Check sheet for the modelled part. Datum: model origin and axes. Units: mm. Round coordinates to 2 decimals unless told otherwise and drop trailing zeros. Order: outer loops, then holes, each group sorted by start corner. A loop starts at its lowest first (then second) coordinate and runs counter-clockwise, first axis right, second up. Notation, with made-up numbers: (64, 78) -> (82, 78) arc R23 cw to (82, 117) -> close; hole circle Ø1 at (-23, 22.25). An arc over 180 degrees is marked (long way). Answer in a Markdown table with one row per item.
```python
from build123d import *

# Parameters (mm, degrees)
FILLET1_R           = 2
FILLET2_R           = 10
SKETCH3_W           = 10
SKETCH3_H           = 20
BOSS_EXTRUDE1_DEPTH = 25
BOSS_EXTRUDE2_REACH = 322.147
SKETCH4_W           = 50
SKETCH4_H           = 20


with BuildPart() as part:
    # Sketch1 → Revolve1 (revolve)
    with BuildSketch(Plane.XY):
        Polygon((0, 0), (150, 0), (50, 100), (25, 100), (25, 50), (0, 50), align=None)
    revolve(axis=Axis((0, 50, 0), (0, -1, 0)))

    # Fillet1
    fillet1_edges = [part.edges().sort_by_distance(p)[0] for p in [
        (-25, 100, 0),
        (-50, 100, 0),
    ]]
    fillet(fillet1_edges, radius=FILLET1_R)

    # Fillet2
    fillet2_edges = [part.edges().sort_by_distance(p)[0] for p in [
        (-150, 0, 0),
    ]]
    fillet(fillet2_edges, radius=FILLET2_R)

    # Sketch4 → Boss-Extrude2 (add, up to next)
    with BuildSketch(Plane(origin=(-136.238585348, 0, 0), x_dir=(0, 0, -1), z_dir=(1, 0, 0)), mode=Mode.PRIVATE) as boss_extrude2_sk1:
        with Locations((0, 15)):
            Rectangle(SKETCH4_W, SKETCH4_H)
    boss_extrude2_tool1 = extrude(boss_extrude2_sk1.sketch, amount=BOSS_EXTRUDE2_REACH, mode=Mode.PRIVATE) - part.part


with BuildPart() as body_2:
    # Sketch3 → Boss-Extrude1 (new, symmetric)
    with BuildSketch(Plane.XY):
        with Locations((-141.238585348, 15)):
            Rectangle(SKETCH3_W, SKETCH3_H)
    extrude(amount=BOSS_EXTRUDE1_DEPTH, both=True)


with BuildPart() as part_1:
    add(part.part)

    add(body_2.part)  # Boss-Extrude2 merges body 2
    add(boss_extrude2_tool1.solids().sort_by_distance((-136.238585, 15, 0))[0])


solid = part_1.part
```
(1) Draft check along X on faces 1 (the flat face through (0, 50, 0)), 2 (the conical face through (52.06, 95.42, 16.4)), 3 (the cylindrical face through (23.846, 73.664, 7.509)), 4 (the flat face through (-139, 5, 0)). Enter one of: pulls with the +X half, pulls with the -X half, needs draft (parallel to the pull), parting line crosses it, or undercut.
Solutions:
| item | result |
|---|---|
| face 1 | undercut |
| face 2 | parting line crosses it |
| face 3 | undercut |
| face 4 | needs draft |
(2) Section check D-D on y = 83. Record the boundary of the cut face in (x, z).
Solutions:
| item | result |
|---|---|
| outline | circle Ø134 at (0, 0); hole circle Ø50 at (0, 0) |
(3) Section check B-B on z = 0. Record the boundary of the cut face in (x, y).
Solutions:
| item | result |
|---|---|
| outline | (-146.24, 5) -> (-134.52, 5) arc R10 ccw to (-125.86, 0) -> (125.86, 0) arc R10 ccw to (132.93, 17.07) -> (50.59, 99.41) arc R2 ccw to (49.17, 100) -> (27, 100) arc R2 ccw to (25, 98) -> (25, 50) -> (-25, 50) -> (-25, 98) arc R2 ccw to (-27, 100) -> (-49.17, 100) arc R2 ccw to (-50.59, 99.41) -> (-125, 25) -> (-146.24, 25) -> close |
(4) Scan lines: probe 1 along Z at (x, y) = (0, 68); probe 2 along Z at (x, y) = (0, 65); probe 3 along Z at (x, y) = (-92.5, 16). Record each from-to range of solid material in increasing order. Write a range as from..to.
Solutions:
| item | result |
|---|---|
| probe 1 | -82..-25, 25..82 |
| probe 2 | -85..-25, 25..85 |
| probe 3 | -96.76..96.76 |
(5) Section check C-C on y = 45.5. Record the boundary of the cut face in (x, z), plus the area to 3 significant figures.
Solutions:
| item | result |
|---|---|
| outline | circle Ø209 at (0, 0) |
| area | 34,300 mm^2 |
(6) Depth check by flat-ended pin: pin 1 Ø11.5 at (x, z) = (-137.5, -1) entering from -Y; pin 2 Ø8 at (x, y) = (46.5, 34.5) entering from -Z; pin 3 Ø1 at (x, z) = (97, -75.5) entering from +Y. Enter the tip coordinate at first touch or a pass-through.
Solutions:
| item | result |
|---|---|
| pin 1 | y = 1.92 |
| pin 2 | z = -110.39 |
| pin 3 | y = 27.58 |
(7) Section check A-A on x = 0. Record the boundary of the cut face in (y, z), plus the area to 3 significant figures.
Solutions:
| item | result |
|---|---|
| outline | (0, -125.86) arc R10 ccw to (17.07, -132.93) -> (99.41, -50.59) arc R2 ccw to (100, -49.17) -> (100, -27) arc R2 ccw to (98, -25) -> (50, -25) -> (50, 25) -> (98, 25) arc R2 ccw to (100, 27) -> (100, 49.17) arc R2 ccw to (99.41, 50.59) -> (17.07, 132.93) arc R10 ccw to (0, 125.86) -> close |
| area | 17,300 mm^2 |
